Here's the drawing with two shaded views (mm, measured from the low corner). I have some questions. A direction names the side the tool comes from. Round coordinates to 2 decimals unless told otherwise and drop trailing zeros. Order: outer loops, then holes, each group sorted by start corner. A loop starts at its lowest first (then second) coordinate and runs counter-clockwise, first axis right, second up.
Q1. If I drill on line 1 (Z direction, x = 15, y = 3.1); line 2 (X direction, y = 26, z = 11.5), over which ranges is the centre line in solid material (lowest first)?
Q2. Will these pins go through, and if not, where does the flat tip stop? P1, Ø4.5, axis at x = 9, y = 28.5, coming from the +Z side; P2, Ø6.5, axis at y = 30, z = 9, coming from the +X side; P3, Ø5.5, axis at x = 16, z = 8.5, coming from the +Y side.
Q3. For the marked faces 1 and 2, which set-ups out of +Z, -Z, +X, -X, +Y, -Y let a thin tool reach every point of the face, with its end or its side?
Q4. If we section it at C-C (x = 30): Please give me the cut outline in (y, z), plus the area to 3 significant figures.
Q5. If we section it at D-D (y = 30): Please give me the cut outline in (x, z), plus the area to 3 significant figures.
Q6. If we section it at A-A (y = 15): Please give me the cut outline in (x, z).
Q7. We'd pull the mould along Z, two halves only. Please class the marked faces 3, 4 and 5: pulls with the +Z half, pulls with the -Z half, needs draft (parallel to the pull), parting line crosses it, or undercut.
Q8. If we section it at B-B (z = 9): Please give me the cut outline in (x, y).
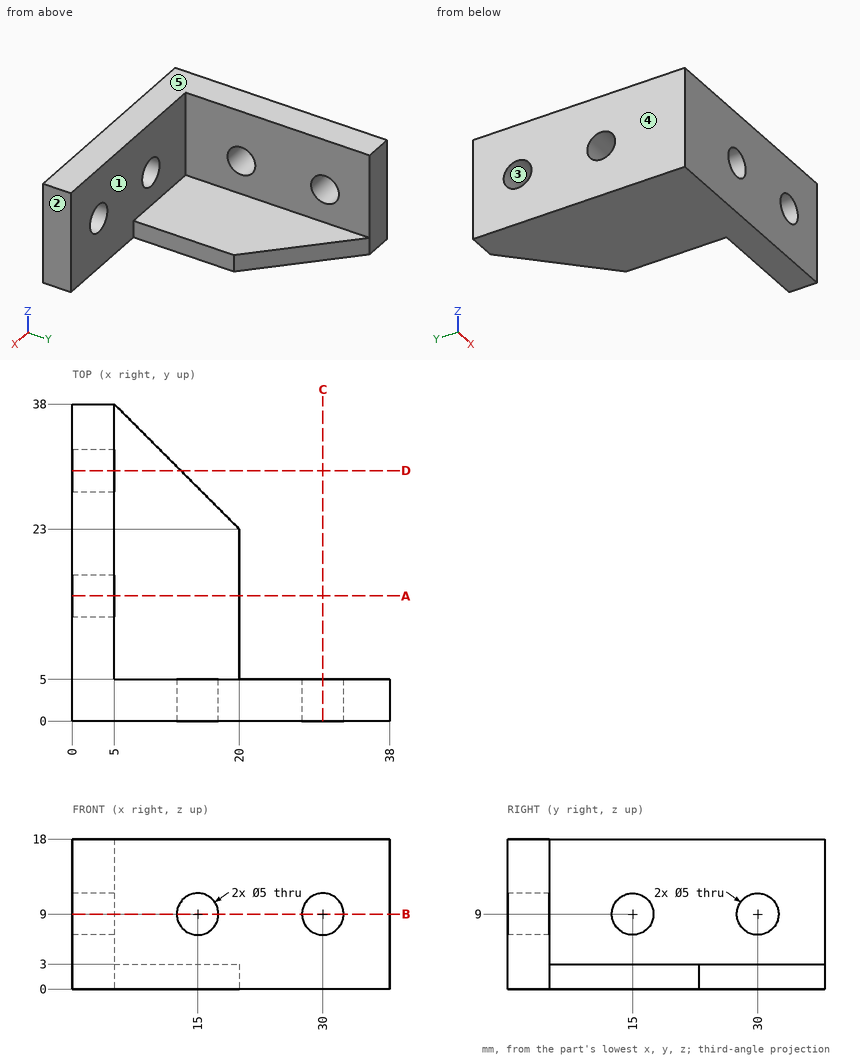
Solution:
1. line 1: z = 0 to 6.5, 11.5 to 18
1. line 2: x = 0 to 5
2. P1: stops at z = 3
2. P2: stops at x = 5
2. P3: stops at y = 5
3. face 1: +Z, +X, +Y
3. face 2: +Z, -Z, +X, +Y, -Y
4. outline: (0, 0) - (5, 0) - (5, 6.5) - (0, 6.5) - close; (0, 11.5) - (5, 11.5) - (5, 18) - (0, 18) - close
4. area: 65.0 mm2
5. outline: (0, 0) - (13, 0) - (13, 3) - (5, 3) - (5, 6.5) - (0, 6.5) - close; (0, 11.5) - (5, 11.5) - (5, 18) - (0, 18) - close
5. area: 89.0 mm2
6. outline: (0, 0) - (20, 0) - (20, 3) - (5, 3) - (5, 6.5) - (0, 6.5) - close; (0, 11.5) - (5, 11.5) - (5, 18) - (0, 18) - close
7. face 3: undercut
7. face 4: needs draft
7. face 5: pulls with the +Z half
8. outline: (0, 0) - (12.5, 0) - (12.5, 5) - (5, 5) - (5, 12.5) - (0, 12.5) - close; (0, 17.5) - (5, 17.5) - (5, 27.5) - (0, 27.5) - close; (0, 32.5) - (5, 32.5) - (5, 38) - (0, 38) - close; (17.5, 0) - (27.5, 0) - (27.5, 5) - (17.5, 5) - close; (32.5, 0) - (38, 0) - (38, 5) - (32.5, 5) - close
